For this review, take the finished solid that the model builds, in its own axes (mm). A direction names the side the tool comes from. Give positions to 0.01 mm unless a question says otherwise; leave off trailing zeros. Write each loop counter-clockwise with the first axis right and the second up, starting at its lowest first coordinate (ties: lowest second). Pieces come first, ordered by that corner, then holes. Notation, with made-up numbers: (44.25, 15.5) -> (98.25, 15.5) arc R26 ccw to (98.25, 48.5) -> close; hole circle Ø6 at (1.25, -2.75). An arc over 180 degrees is marked (long way). Return JSON: item names as keys, results as strings.
from build123d import *

# Parameters (mm, degrees)
F0_W     = 8.89
F0_H     = 3.175
F0_W_2   = 9.144
F1_DEPTH = 3.175
F2_R     = 3.9878
F2_R_2   = 4.4958
F3_DEPTH = 25.4


with BuildPart() as f1:
    # F0 (on Top) → F1 (new body)
    with BuildSketch(Plane.XY):
        with Locations((-25.0698, 16.8275)):
            Rectangle(F0_W, F0_H)
        Polygon((-29.5148, 15.24), (-38.1, 15.24), (-38.1, -15.24), (-29.5148, -15.24), (-29.5148, -12.065), (-20.6248, -12.065), (-20.6248, -15.24), (-4.572, -15.24), (-4.572, -12.065), (4.572, -12.065), (4.572, -15.24), (20.6248, -15.24), (20.6248, -12.065), (29.5148, -12.065), (29.5148, -15.24), (38.1, -15.24), (38.1, 15.24), (29.5148, 15.24), (20.6248, 15.24), (4.572, 15.24), (-4.572, 15.24), (-20.6248, 15.24), align=None)
        with Locations((0, 16.8275)):
            Rectangle(F0_W_2, F0_H)
        with Locations((25.0698, 16.8275)):
            Rectangle(F0_W, F0_H)
    extrude(amount=F1_DEPTH)

    # F2 (on face) → F3 (cut)
    with BuildSketch(Plane.XY.offset(3.175)):
        with Locations((-12.8858196329, 0)):
            Circle(F2_R)
        with Locations((10.5130393058, 0)):
            Circle(F2_R_2)
        with Locations((23.2130393058, 0)):
            Circle(F2_R_2)
    extrude(amount=-F3_DEPTH, mode=Mode.SUBTRACT)


solid = f1.part
1. Add section A-A, the plane y = 0. State the section outline as (x, z) points (3 decimals), plus the area to 3 significant figures.
Results found:
{"outline": "(-38.1, 0) -> (-16.874, 0) -> (-16.874, 3.175) -> (-38.1, 3.175) -> close; (-8.898, 0) -> (6.017, 0) -> (6.017, 3.175) -> (-8.898, 3.175) -> close; (15.009, 0) -> (18.717, 0) -> (18.717, 3.175) -> (15.009, 3.175) -> close; (27.709, 0) -> (38.1, 0) -> (38.1, 3.175) -> (27.709, 3.175) -> close", "area": "160 mm²"}
2. To check wall thickness, follow probe 1 along X at (y, z) = (15.5, 1.1); probe 2 along X at (y, z) = (3.5, 0.75); probe 3 along X at (y, z) = (-2, 2.45). State the ranges of each line that lie inside material, in increasing order.
Results found:
{"probe 1": "x = -29.51 to -20.62, -4.57 to 4.57, 20.62 to 29.51", "probe 2": "x = -38.1 to -14.8, -10.97 to 7.69, 13.33 to 20.39, 26.03 to 38.1", "probe 3": "x = -38.1 to -16.34, -9.44 to 6.49, 14.54 to 19.19, 27.24 to 38.1"}
3. Add section B-B, the plane z = 1.4. Count the separate pieces of the cut face and the enclosed holes in it, plus the area to 3 significant figures.
Results found:
{"separate pieces": "1", "enclosed holes": "3", "area": "2,150 mm²"}
4. For pin 1 (1 mm diameter, centred on x = -32.5, z = 2, fed in from +Y); pin 2 (1 mm diameter, centred on y = 17.5, z = 2, fed in from +X); pin 3 (1.6 mm diameter, centred on y = 17, z = 1.5, fed in from -X), all flat-tipped, find the tip position at first contact; note any pin that passes through.
Results found:
{"pin 1": "stops at y = 15.24", "pin 2": "stops at x = 29.51", "pin 3": "stops at x = -29.51"}
5. Add section C-C, the plane x = -33. State the section outline as (y, z) points (3 decimals).
Results found:
{"outline": "(-15.24, 0) -> (15.24, 0) -> (15.24, 3.175) -> (-15.24, 3.175) -> close"}
6. For faces 1 (the flat face through (-4.572, 17, 2)), 2 (the flat face through (-1, 2, 0)), 3 (the flat face through (34, 15.24, 2)), 4 (the cylindrical face through (6.02, 0.2, 1.61)), 5 (the flat face through (-29.515, -14, 2)), list the 3-axis set-ups (+Z, -Z, +X, -X, +Y, -Y) from which the entire face can be reached by the end or side of a thin tool; tool diameter is ignored.
Results found:
{"face 1": "+Z, -Z, +Y", "face 2": "-Z, +X, -X, +Y, -Y", "face 3": "+Z, -Z, +X, +Y", "face 4": "+Z, -Z", "face 5": "+Z, -Z, -Y"}
7. The part is to be moulded in two halves that separate along X. For faces 6 (the flat face through (0, 18.415, 2)), 7 (the flat face through (-38.1, 0, 2)), 8 (the flat face through (20.625, -14, 2)), say which applies: +X half, -X half, draft (parallel to the pull), parting line (faces both ways), or undercut.
Results found:
{"face 6": "draft", "face 7": "-X half", "face 8": "undercut"}
